Design review of the part built by this model. Coordinates are the model's own, in mm. A direction names the side the tool comes from. Give positions to 0.01 mm unless a question says otherwise; leave off trailing zeros. Loops run counter-clockwise (first coordinate to the right, second up) from the corner with the lowest first, then second, coordinate; pieces in that order, holes last.
Autodesk Inventor part; units mm, degrees
ref_plane "YZ Plane" through (0, 0, 0) normal (1, 0, 0) x (0, 1, 0)
ref_plane "XZ Plane" through (0, 0, 0) normal (0, 1, 0) x (-1, 0, 0)
ref_plane "XY Plane" through (0, 0, 0) normal (0, 0, 1) x (1, 0, 0)
sketch "Sketch1" plane through (0, 0, 0) normal (0, 0, 1) x (1, 0, 0)
  line L0 (0, 0) -> (15.875, 0)
  line L1 (15.875, 0) -> (15.875, 0.7937)
  line L2 (15.875, 0.7937) -> (0.7938, 0.7937)
  line L3 (0.7938, 0.7937) -> (0.7937, 15.875)
  line L4 (0.7937, 15.875) -> (0, 15.875)
  line L5 (0, 15.875) -> (0, 0)
  dimension "d0" = 15.875
  dimension "d1" = 0.7937
  dimension "d2" = 0.7937
extrude "Extrusion1" add sketch "Sketch1" along normal blind 474.6752
sketch "Sketch2" plane through (0.7937, 0.7937, 0) normal (1, 0, 0) x (0, 0, -1)
  line L0 (0, 0) -> (0, 15.0812)
  line L1 (-474.6752, 0) -> (-474.6752, 15.0812)
  circle A0 centre (-19.0627, 7.5406) radius 2.2479
  circle A1 centre (-63.5127, 7.5406) radius 2.2479
  line L2 (0, 7.5406) -> (-474.6752, 7.5406) construction
  circle A2 centre (-6.35, 7.5406) radius 2.2479
  circle A3 centre (-82.55, 7.5406) radius 2.2479
  circle A4 centre (-246.0752, 7.5406) radius 2.2479
  circle A5 centre (-455.6252, 7.5406) radius 2.2479
  circle A6 centre (-347.6752, 7.5406) radius 2.2479
  circle A7 centre (-369.6843, 8.0867) radius 1.905
  point P0 (0, -0.7937)
  dimension "d5" = 4.4958
  dimension "d8" = 19.05
  dimension "d9" = 127
  dimension "d10" = 228.6
  dimension "d11" = 6.35
  dimension "d12" = 82.55
extrude "Extrusion2" cut sketch "Sketch2" against normal through all
properties part number "Electrical Board 1 Bracing L Channel" material "Aluminum 6061"
Q1. Take a section at B-B (x = 5). Give the boundary of the cut face in (y, z), plus the area to 3 significant figures.
Results:
outline: (0, 0) - (0.79, 0) - (0.79, 474.68) - (0, 474.68) - close
area: 377 mm2
Q2. Insertion check: pin 1 (5 mm diameter, centred on y = 8.33, z = 455.63, fed in from +X); pin 2 (7 mm diameter, centred on y = 8.33, z = 63.51, fed in from -X); pin 3 (4.5 mm diameter, centred on x = 5.5, z = 255, fed in from +Y). Each pin has a flat end and moves straight along its axis. Give the tip position at first contact, or say it passes through.
Results:
pin 1: stops at x = 0.79
pin 2: stops at x = 0
pin 3: stops at y = 0.79
Q3. Wall thickness on line 1 (Y direction, x = 0.5, z = 82.55) (3 decimals); line 2 (X direction, y = 6.25, z = 126): over which ranges is each line inside the solid? List them lowest first.
Results:
line 1: y = 0 to 6.086, 10.582 to 15.875
line 2: x = 0 to 0.79
Q4. Take a section at A-A (z = 104). Give the boundary of the cut face in (x, y) (3 decimals).
Results:
outline: (0, 0) - (15.875, 0) - (15.875, 0.794) - (0.794, 0.794) - (0.794, 15.875) - (0, 15.875) - close
Q5. Tool access review of faces 1 (the face through (4.4, 0.3, 474.675)), 2 (the face through (8, 0.794, 234)): name each direction out of +Z, -Z, +X, -X, +Y, -Y from which nothing blocks a thin tool from reaching the whole face with its end or side.
Results:
face 1: +Z, +X, -X, +Y, -Y
face 2: +Z, -Z, +X, +Y
